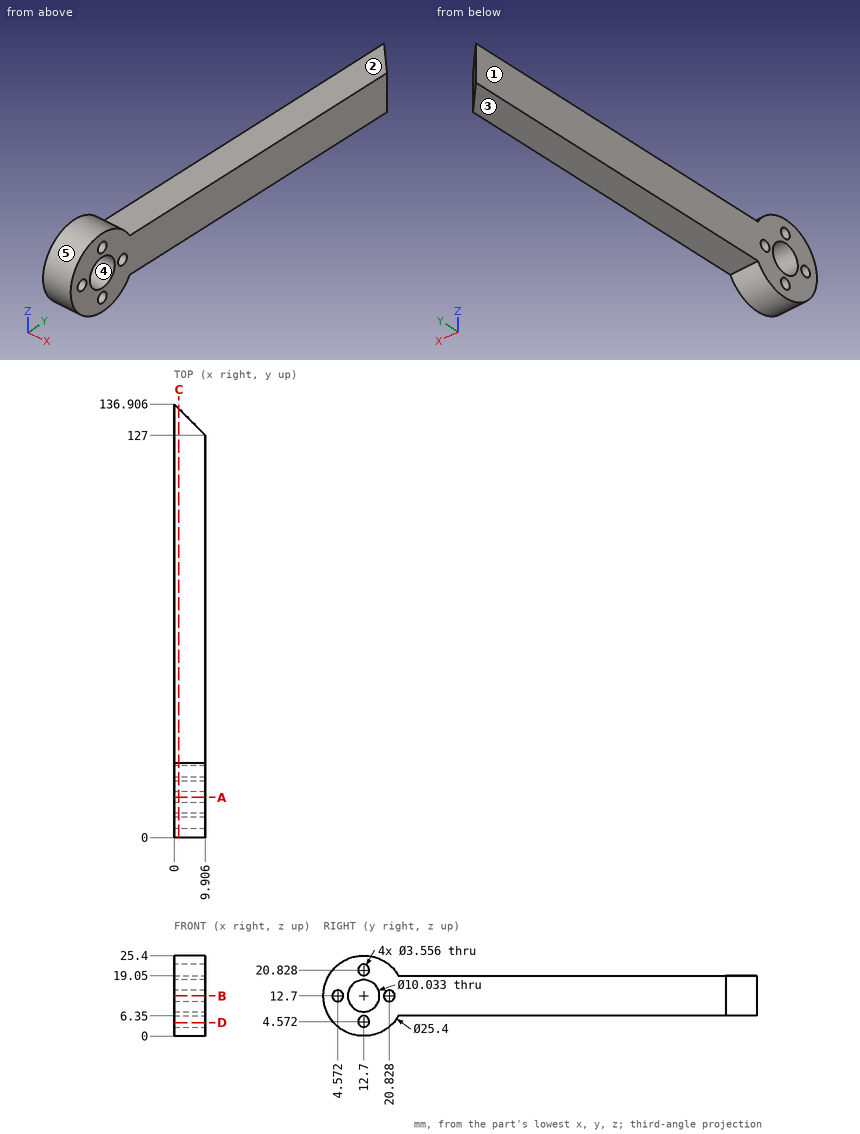
Geometry check sheet. Reference: drawing and pictorial views, mm from the part's lowest x, y, z. A direction names the side the tool comes from. Coordinates: 2 decimals unless noted, no trailing zeros. Loops run counter-clockwise (first coordinate to the right, second up) from the corner with the lowest first, then second, coordinate; pieces in that order, holes last. Notation, with made-up numbers: (87.25, -20) -> (99.25, -20) arc R28 ccw to (99.25, 18) -> close; hole circle Ø11 at (83, 41). An arc over 180 degrees is marked (long way). Put each result on its own line as item: value.
1) Gauge pin test, flat ends, axial feed: pin 1 Ø5.5 at (y, z) = (12.7, 20.828) entering from +X; pin 2 Ø3 at (x, y) = (5.5, 46) entering from +Z; pin 3 Ø2 at (y, z) = (4.572, 12.7) entering from -X; pin 4 Ø3 at (x, z) = (2.5, 22.5) entering from -Y. Record the tip position at first contact, or that the pin passes through.
Result set:
pin 1: stops at x = 9.91
pin 2: stops at z = 19.05
pin 3: passes through
pin 4: stops at y = 3.09
2) Cross-section at C-C on x = 1.5. Record the boundary of the cut face in (y, z).
Result set:
outline: (23.7, 6.35) -> (135.41, 6.35) -> (135.41, 19.05) -> (23.7, 19.05) arc R12.7 ccw (long way) to start; hole circle Ø3.56 at (4.57, 12.7); hole circle Ø10.03 at (12.7, 12.7); hole circle Ø3.56 at (12.7, 4.57); hole circle Ø3.56 at (12.7, 20.83); hole circle Ø3.56 at (20.83, 12.7)
3) Cross-section at D-D on z = 4.25. Record the boundary of the cut face in (x, y).
Result set:
outline: (0, 3.22) -> (9.91, 3.22) -> (9.91, 10.95) -> (0, 10.95) -> close; (0, 14.45) -> (9.91, 14.45) -> (9.91, 22.18) -> (0, 22.18) -> close
4) Tool access check on the marked faces 1 and 2. Record the directions out of +Z, -Z, +X, -X, +Y, -Y that give a thin tool (end or side, any length) a straight path to the whole face; none if there is none.
Result set:
face 1: +Z, -Z, -X, +Y, -Y
face 2: +Z, +X, -X, +Y
5) Cross-section at B-B on z = 12.7. Record the boundary of the cut face in (x, y).
Result set:
outline: (0, 0) -> (9.91, 0) -> (9.91, 2.79) -> (0, 2.79) -> close; (0, 6.35) -> (9.91, 6.35) -> (9.91, 7.68) -> (0, 7.68) -> close; (0, 17.72) -> (9.91, 17.72) -> (9.91, 19.05) -> (0, 19.05) -> close; (0, 22.61) -> (9.91, 22.61) -> (9.91, 127) -> (0, 136.91) -> close
6) Thickness scan on line 1 (Y direction, x = 6.5, z = 12.7); line 2 (Y direction, x = 7.25, z = 12.7); line 3 (Z direction, x = 9.5, y = 14). Record the ranges inside material, lowest first.
Result set:
line 1: y = 0 to 2.79, 6.35 to 7.68, 17.72 to 19.05, 22.61 to 130.41
line 2: y = 0 to 2.79, 6.35 to 7.68, 17.72 to 19.05, 22.61 to 129.66
line 3: z = 0.07 to 3.36, 5.78 to 7.85, 17.55 to 19.62, 22.04 to 25.33
7) Release check for a two-part mould opening along Y. For the marked faces 3, 4 and 5 record: released by +Y, released by -Y, zero draft, split by the parting line, or undercut.
Result set:
face 3: zero draft
face 4: undercut
face 5: split by the parting line
8) Cross-section at A-A on y = 12.7. Record the boundary of the cut face in (x, z), plus the area to 3 significant figures.
Result set:
outline: (0, 0) -> (9.91, 0) -> (9.91, 2.79) -> (0, 2.79) -> close; (0, 6.35) -> (9.91, 6.35) -> (9.91, 7.68) -> (0, 7.68) -> close; (0, 17.72) -> (9.91, 17.72) -> (9.91, 19.05) -> (0, 19.05) -> close; (0, 22.61) -> (9.91, 22.61) -> (9.91, 25.4) -> (0, 25.4) -> close
area: 81.8 mm^2
